Input: dimensioned drawing with shaded views. Units: mm. Origin: part minimum x, y, z. Give positions to 0.01 mm unless a question says otherwise; leave off trailing zeros. Loops run counter-clockwise (first coordinate to the right, second up) from the corner with the lowest first, then second, coordinate; pieces in that order, holes last. Notation, with made-up numbers: (-36, 1) -> (23, 1) arc R18 cw to (23, 5) -> close; hole circle Ø11 at (-14.5, 20.5). An arc over 180 degrees is marked (long way). Answer as a JSON object with one key per item and string values.
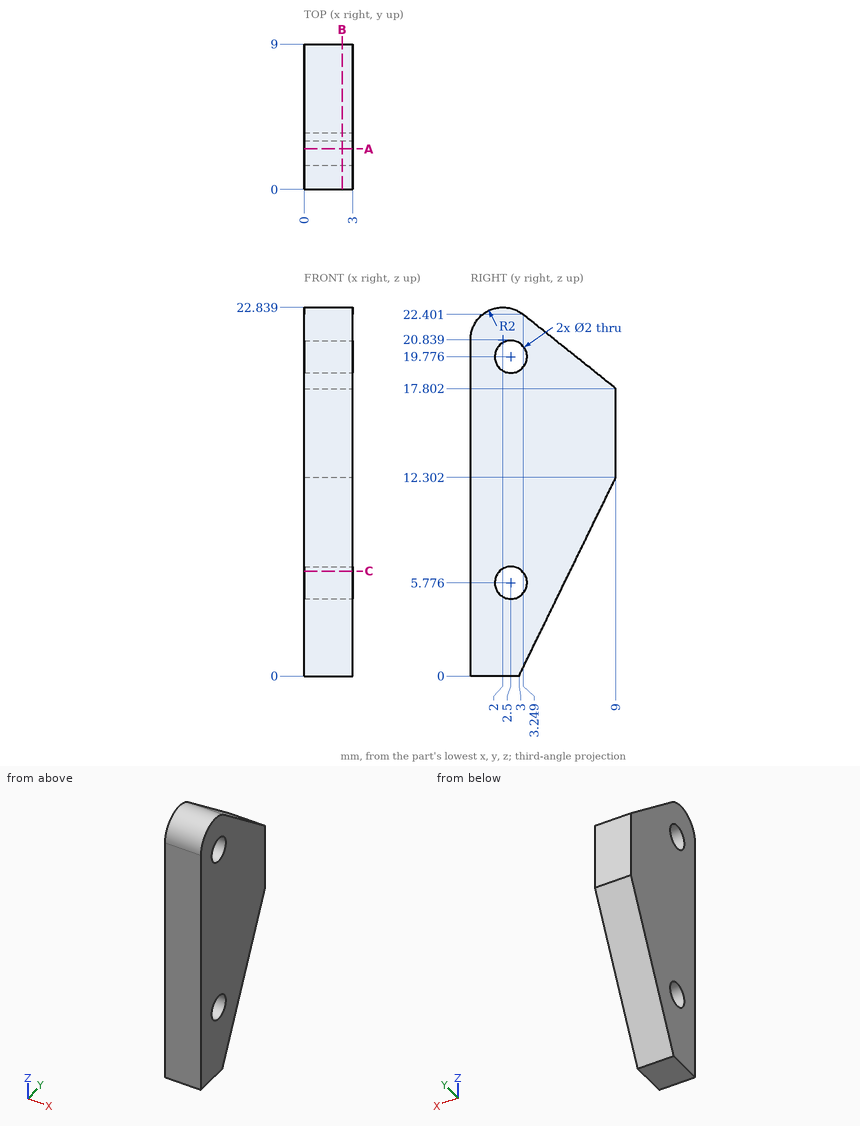
Q1. Section B-B, the plane x = 2.35. Return the cut outline in (y, z), then the cut area to 3 significant figures.
Evaluation:
{"outline": "(0, 0) -> (3, 0) -> (9, 12.3) -> (9, 17.8) -> (3.25, 22.4) arc R2 ccw to (0, 20.84) -> close; hole circle Ø2 at (2.5, 5.78); hole circle Ø2 at (2.5, 19.78)", "area": "146 mm2"}
Q2. Section A-A, the plane y = 2.5. Return the cut outline in (x, z).
Evaluation:
{"outline": "(0, 0) -> (3, 0) -> (3, 4.78) -> (0, 4.78) -> close; (0, 6.78) -> (3, 6.78) -> (3, 18.78) -> (0, 18.78) -> close; (0, 20.78) -> (3, 20.78) -> (3, 22.78) -> (0, 22.78) -> close"}
Q3. Pin query (flat end, axial travel): pin 1 (1.8 mm diameter, centred on y = 2.5, z = 5.78, fed in from +X); pin 2 (1.5 mm diameter, centred on x = 1.5, y = 6, fed in from -Z) (1 decimal). Return the tip coordinate at first contact, or that it passes through.
Evaluation:
{"pin 1": "passes through", "pin 2": "stops at z = 4.6"}
Q4. Ray query, line 1 along Z through (x, y) = (0.75, 2.5) (1 decimal); line 2 along Z through (x, y) = (0.5, 2); line 3 along Y through (x, z) = (2.9, 3). Return the intervals inside material, ascending.
Evaluation:
{"line 1": "z = 0 to 4.8, 6.8 to 18.8, 20.8 to 22.8", "line 2": "z = 0 to 4.91, 6.64 to 18.91, 20.64 to 22.84", "line 3": "y = 0 to 4.46"}
Q5. Section C-C, the plane z = 6.5. Return the cut outline in (x, y).
Evaluation:
{"outline": "(0, 0) -> (3, 0) -> (3, 1.81) -> (0, 1.81) -> close; (0, 3.19) -> (3, 3.19) -> (3, 6.17) -> (0, 6.17) -> close"}
